from build123d import *

# Parameters (mm, degrees)
F1_DEPTH = 568.325
F2_R     = 2.38125
F3_DEPTH = 3.175
F4_R     = 2.38125
F5_DEPTH = 3.175
F7_DEPTH = 3.175
F9_DEPTH = 35.56


with BuildPart() as f1:
    # F0 (on Top) → F1 (new body)
    with BuildSketch(Plane.XY):
        Polygon((0, 25.4), (0, 0), (25.4, 0), (25.4, 3.175), (3.175, 3.175), (3.175, 25.4), align=None)
    extrude(amount=F1_DEPTH)

    # F2 (on face) → F3 (cut)
    with BuildSketch(Plane(origin=(0, 0, 0), x_dir=(0, -1, 0), z_dir=(-1, 0, 0))):
        with Locations((-15.875, 517.525)):
            Circle(F2_R)
        with Locations((-15.875, 212.725)):
            Circle(F2_R)
    extrude(amount=-F3_DEPTH, mode=Mode.SUBTRACT)

    # F4 (on face) → F5 (cut)
    with BuildSketch(Plane.XZ):
        with Locations((15.875, 458.7875)):
            Circle(F4_R)
        with Locations((15.875, 106.3625)):
            Circle(F4_R)
        with Locations((15.875, 539.75)):
            Circle(F4_R)
    extrude(amount=-F5_DEPTH, mode=Mode.SUBTRACT)

    # F6 (on face) → F7 (cut)
    with BuildSketch(Plane(origin=(0, 0, 0), x_dir=(0, -1, 0), z_dir=(-1, 0, 0))):
        Polygon((-25.4, 0), (-4.7625, 0), (-4.7625, 38.1), (-25.4, 46.4380912357), align=None)
    extrude(amount=-F7_DEPTH, mode=Mode.SUBTRACT)

    # F8 (on face) → F9 (join)
    with BuildSketch(Plane(origin=(0, 0, 0), x_dir=(1, 0, 0), z_dir=(0, 0, -1))):
        with BuildLine():
            ThreePointArc((13.0437542426, -9.5063361704), (12.8721302689, -9.520330609), (12.7, -9.525))
            Line((12.7, -9.525), (12.7, -12.7))
            ThreePointArc((12.7, -12.7), (13.0442605378, -12.6906612181), (13.3875084853, -12.6626723408))
            ThreePointArc((13.3875084853, -12.6626723408), (19.5337619369, -10.8104975605), (24.6005143968, -6.8690508185))
            Line((24.6005143968, -6.8690508185), (22.225, -4.7625))
            ThreePointArc((22.225, -4.7625), (18.0763265852, -7.9897694283), (13.0437542426, -9.5063361704))
        make_face()
        with BuildLine():
            ThreePointArc((12.7, -9.525), (12.5278697311, -9.520330609), (12.3562457574, -9.5063361704))
            ThreePointArc((12.3562457574, -9.5063361704), (7.3236734148, -7.9897694283), (3.175, -4.7625))
            Line((3.175, -4.7625), (0, -4.7625))
            ThreePointArc((0, -4.7625), (0.2065927495, -5.8890803989), (0.7994856032, -6.8690508185))
            ThreePointArc((0.7994856032, -6.8690508185), (5.8662380631, -10.8104975605), (12.0124915147, -12.6626723408))
            ThreePointArc((12.0124915147, -12.6626723408), (12.3557394622, -12.6906612181), (12.7, -12.7))
            Line((12.7, -12.7), (12.7, -9.525))
        make_face()
    extrude(amount=-F9_DEPTH)


solid = f1.part
Could you check a few things on this model? Use its own coordinates, in mm. A direction names the side the tool comes from. Coordinates: 2 decimals unless noted, no trailing zeros. Loops run counter-clockwise (first coordinate to the right, second up) from the corner with the lowest first, then second, coordinate; pieces in that order, holes last. Notation, with made-up numbers: (10.25, -34.75) -> (47.25, -34.75) arc R20 ccw to (47.25, -19.75) -> close; hole circle Ø10 at (-7.5, 5). An arc over 180 degrees is marked (long way). Answer in a Markdown table with one row per item.
(1) Will these pins go through, and if not, where does the flat tip stop? pin 1 Ø6 at (x, z) = (16.5, 280.5) entering from +Y (3 decimals); pin 2 Ø4 at (x, y) = (6.5, 8.5) entering from +Z; pin 3 Ø6.5 at (y, z) = (18.5, 397.5) entering from +X (3 decimals).
Results found:
| item | result |
|---|---|
| pin 1 | stops at y = 3.175 |
| pin 2 | stops at z = 35.56 |
| pin 3 | stops at x = 3.175 |
(2) Thinking about a two-plate mould opening in Y: for faces 1 (the face through (7.39, 8.024, 17.531)), 2 (the face through (13, 0, 280)), 3 (the face through (0, 13, 280)), which applies, released by +Y, released by -Y, zero draft, split by the parting line, or undercut?
Results found:
| item | result |
|---|---|
| face 1 | undercut |
| face 2 | released by -Y |
| face 3 | zero draft |
(3) Imagine slicing it at A-A (z = 423). List the corners of the cut face in (x, y) for me (3 decimals), plus the area to 3 significant figures.
Results found:
| item | result |
|---|---|
| outline | (0, 0) -> (25.4, 0) -> (25.4, 3.175) -> (3.175, 3.175) -> (3.175, 25.4) -> (0, 25.4) -> close |
| area | 151 mm^2 |
(4) If I drill on probe 1 along X at (y, z) = (1.85, 539.75); probe 2 along X at (y, z) = (6, 380.5) (3 decimals), over which ranges is the centre line in solid material (lowest first)?
Results found:
| item | result |
|---|---|
| probe 1 | x = 0 to 13.49, 18.26 to 25.4 |
| probe 2 | x = 0 to 3.175 |
(5) For faces 4 (the face through (18.142, 7.956, 17.531)), 5 (the face through (5.79, 10.77, 17.53)), 6 (the face through (7, 2, 568.325)), which set-ups out of +Z, -Z, +X, -X, +Y, -Y let a thin tool reach every point of the face, with its end or its side?
Results found:
| item | result |
|---|---|
| face 4 | +Z, -Z |
| face 5 | -Z, -X, +Y |
| face 6 | +Z, +X, -X, +Y, -Y |
